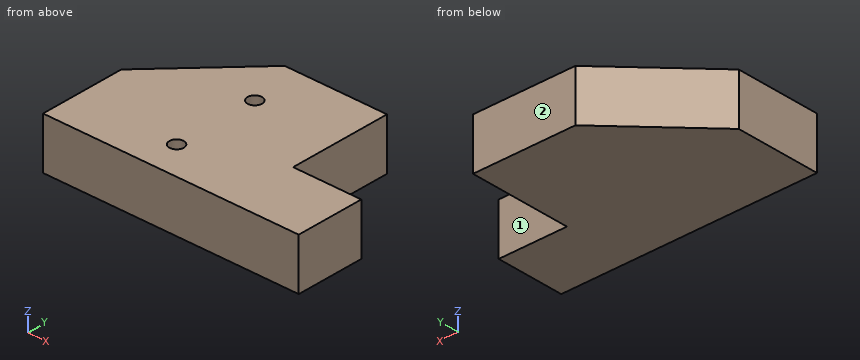
```python
from build123d import *

# Parameters (mm, degrees)
SALIENTE_EXTRUIR1_DEPTH            = 30
TALADRO_DE_MARGEN_PARA_5_161_D     = 8.4328
TALADRO_DE_MARGEN_PARA_5_161_DEPTH = 25.4
TALADRO_DE_MARGEN_PARA_5_161_TIP   = 2.533468714


with BuildPart() as part:
    # Croquis1 → Saliente-Extruir1 (new body)
    with BuildSketch(Plane.XY):
        Polygon((0, 0), (0, 50), (50, 100), (110, 100), (110, 40), (150, 40), (150, 0), align=None)
    extrude(amount=SALIENTE_EXTRUIR1_DEPTH)

    # Taladro de margen para 5/161
    with Locations(Plane(origin=(60, 70, 30), x_dir=(1, 0, 0), z_dir=(0, 0, 1))):
        with Locations((0, 0), (0, -50)):
            Hole(TALADRO_DE_MARGEN_PARA_5_161_D / 2, depth=TALADRO_DE_MARGEN_PARA_5_161_DEPTH)
            with Locations((0, 0, -(TALADRO_DE_MARGEN_PARA_5_161_DEPTH + TALADRO_DE_MARGEN_PARA_5_161_TIP / 2))):  # 118° drill point
                Cone(0, TALADRO_DE_MARGEN_PARA_5_161_D / 2, TALADRO_DE_MARGEN_PARA_5_161_TIP, mode=Mode.SUBTRACT)


solid = part.part
```
For this review, take the finished solid that the model builds, in its own axes (mm). Face numbers are marked on the shaded views. A direction names the side the tool comes from. Coordinates: 2 decimals unless noted, no trailing zeros. Write each loop counter-clockwise with the first axis right and the second up, starting at its lowest first coordinate (ties: lowest second). Pieces come first, ordered by that corner, then holes. Notation, with made-up numbers: (-18.5, 30) - (20.5, 30) arc R23 ccw to (20.5, 39) - close; hole circle Ø5 at (69, -2). An arc over 180 degrees is marked (long way). Answer in a Markdown table with one row per item. Add a question column.
Q1. We need section A-A, the plane z = 22.5. State the section outline as (x, y) points.
Q2. For P1, Ø5, axis at x = 44.5, z = 24.5, coming from the +Y side; P2, Ø15, axis at x = 136.5, z = 11, coming from the +Y side, all flat-tipped, find the tip position at first contact; note any pin that passes through.
Q3. Tool access review of the marked faces 1 and 2: name each direction out of +Z, -Z, +X, -X, +Y, -Y from which nothing blocks a thin tool from reaching the whole face with its end or side.
Q4. We need section B-B, the plane x = 45. State the section outline as (y, z) points, and give its area (3 significant figures).
Q5. We need section C-C, the plane y = 58. State the section outline as (x, z) points, and give its area (3 significant figures).
Q6. For probe 1 along Y at (x, z) = (60, 22.25); probe 2 along X at (y, z) = (20, 24); probe 3 along Y at (x, z) = (62, 11.5), list the stretches that pass through material, from the lowest coordinate up.
Answer list:
| question | item | result |
|---|---|---|
| 1 | outline | (0, 0) - (150, 0) - (150, 40) - (110, 40) - (110, 100) - (50, 100) - (0, 50) - close; hole circle Ø8.43 at (60, 20); hole circle Ø8.43 at (60, 70) |
| 2 | P1 | stops at y = 97 |
| 2 | P2 | stops at y = 40 |
| 3 | face 1 | +Z, -Z, +X, +Y |
| 3 | face 2 | +Z, -Z, +X, -X, +Y |
| 4 | outline | (0, 0) - (95, 0) - (95, 30) - (0, 30) - close |
| 4 | area | 2,850 mm2 |
| 5 | outline | (8, 0) - (110, 0) - (110, 30) - (8, 30) - close |
| 5 | area | 3,060 mm2 |
| 6 | probe 1 | y = 0 to 15.78, 24.22 to 65.78, 74.22 to 100 |
| 6 | probe 2 | x = 0 to 55.78, 64.22 to 150 |
| 6 | probe 3 | y = 0 to 16.29, 23.71 to 66.29, 73.71 to 100 |
